from build123d import *

# Parameters (mm, degrees)
SKETCH1_R           = 2.125
SKETCH1_R_2         = 3
SKETCH1_W           = 6.35
SKETCH1_H           = 6
SKETCH1_W_2         = 12.7
SKETCH1_H_2         = 5.9944
SKETCH1_H_3         = 6.35
BOSS_EXTRUDE1_DEPTH = 5.9944


with BuildPart() as part:
    # Sketch1 → Boss-Extrude1 (new body)
    with BuildSketch(Plane(origin=(0, 0, 0), x_dir=(-1, 0, 0), z_dir=(0, 0, 1))):
        with BuildLine():
            Line((70.702589937, 1.66614002), (72.098749997, 1.66614002))
            Line((72.098749997, 1.66614002), (72.098749997, 7.383354962))
            Line((72.098749997, 7.383354962), (65.748749997, 7.383354962))
            Line((65.748749997, 7.383354962), (65.748749997, 13.383354962))
            Line((65.748749997, 13.383354962), (72.098749997, 13.383354962))
            Line((72.098749997, 13.383354962), (72.098749997, 45.072109768))
            ThreePointArc((72.098749997, 45.072109768), (69.866903669, 50.460263441), (64.478749997, 52.692109768))
            Line((64.478749997, 52.692109768), (45.302589937, 52.692109768))
            Line((45.302589937, 52.692109768), (19.902589937, 52.692109768))
            Line((19.902589937, 52.692109768), (-35.623445702, 52.692109768))
            ThreePointArc((-35.623445702, 52.692109768), (-40.113573763, 50.832237829), (-41.973445702, 46.342109768))
            Line((-41.973445702, 46.342109768), (-41.973445702, -49.004229729))
            ThreePointArc((-41.973445702, -49.004229729), (-40.113573763, -53.494357789), (-35.623445702, -55.354229729))
            Line((-35.623445702, -55.354229729), (19.902589937, -55.354229729))
            Line((19.902589937, -55.354229729), (45.302589937, -55.354229729))
            Line((45.302589937, -55.354229729), (64.478749997, -55.354229729))
            ThreePointArc((64.478749997, -55.354229729), (69.866903669, -53.122383402), (72.098749997, -47.734229729))
            Line((72.098749997, -47.734229729), (72.098749997, -12.840645038))
            Line((72.098749997, -12.840645038), (65.748749997, -12.840645038))
            Line((65.748749997, -12.840645038), (65.748749997, -6.840645038))
            Line((65.748749997, -6.840645038), (72.098749997, -6.840645038))
            Line((72.098749997, -6.840645038), (72.098749997, -4.32825998))
            Line((72.098749997, -4.32825998), (70.702589937, -4.32825998))
            Line((70.702589937, -4.32825998), (65.829579937, -4.32825998))
            Line((65.829579937, -4.32825998), (65.829579937, 1.66614002))
            Line((65.829579937, 1.66614002), (70.702589937, 1.66614002))
        make_face()
        with Locations((-10.170420063, -18.840645038)):
            Circle(SKETCH1_R, mode=Mode.SUBTRACT)
        with Locations((66.848749997, -36.840645038)):
            Circle(SKETCH1_R, mode=Mode.SUBTRACT)
        with Locations((42.848749997, -18.840645038)):
            Circle(SKETCH1_R, mode=Mode.SUBTRACT)
        with Locations((-28.770420063, -43.34064498)):
            Circle(SKETCH1_R_2, mode=Mode.SUBTRACT)
        with Locations((-28.770420063, -12.34064498)):
            Circle(SKETCH1_R_2, mode=Mode.SUBTRACT)
        with Locations((13.829579937, -18.840645038)):
            Circle(SKETCH1_R, mode=Mode.SUBTRACT)
        with Locations((42.848749997, -36.840645038)):
            Circle(SKETCH1_R, mode=Mode.SUBTRACT)
        with Locations((-10.170420063, -36.840645038)):
            Circle(SKETCH1_R, mode=Mode.SUBTRACT)
        with Locations((66.848749997, -18.840645038)):
            Circle(SKETCH1_R, mode=Mode.SUBTRACT)
        with Locations((13.829579937, -36.840645038)):
            Circle(SKETCH1_R, mode=Mode.SUBTRACT)
        with Locations((-28.770420063, 9.67852502)):
            Circle(SKETCH1_R_2, mode=Mode.SUBTRACT)
        with Locations((-28.770420063, 40.67852502)):
            Circle(SKETCH1_R_2, mode=Mode.SUBTRACT)
        with Locations((-10.170420063, 34.178525078)):
            Circle(SKETCH1_R, mode=Mode.SUBTRACT)
        with Locations((13.829579937, 34.178525078)):
            Circle(SKETCH1_R, mode=Mode.SUBTRACT)
        with Locations((13.829579937, 16.178525078)):
            Circle(SKETCH1_R, mode=Mode.SUBTRACT)
        with Locations((-10.170420063, 16.178525078)):
            Circle(SKETCH1_R, mode=Mode.SUBTRACT)
        with Locations((42.848749997, 34.178525078)):
            Circle(SKETCH1_R, mode=Mode.SUBTRACT)
        with Locations((66.848749997, 34.178525078)):
            Circle(SKETCH1_R, mode=Mode.SUBTRACT)
        with Locations((66.848749997, 16.178525078)):
            Circle(SKETCH1_R, mode=Mode.SUBTRACT)
        with Locations((42.848749997, 16.178525078)):
            Circle(SKETCH1_R, mode=Mode.SUBTRACT)
        with Locations((49.873749997, 10.383354962)):
            Rectangle(SKETCH1_W, SKETCH1_H, mode=Mode.SUBTRACT)
        with Locations((-29.420420063, -1.33105998)):
            Rectangle(SKETCH1_W_2, SKETCH1_H_2, mode=Mode.SUBTRACT)
        with Locations((49.873749997, -9.840645038)):
            Rectangle(SKETCH1_W, SKETCH1_H, mode=Mode.SUBTRACT)
        with Locations((-4.020420063, -1.33105998)):
            Rectangle(SKETCH1_W_2, SKETCH1_H_2, mode=Mode.SUBTRACT)
        with Locations((21.379579937, -1.33105998)):
            Rectangle(SKETCH1_W_2, SKETCH1_H_2, mode=Mode.SUBTRACT)
        with Locations((46.779579937, -1.33105998)):
            Rectangle(SKETCH1_W_2, SKETCH1_H_2, mode=Mode.SUBTRACT)
        with Locations((18.204579937, 5.84394002)):
            Rectangle(SKETCH1_W, SKETCH1_H_3, mode=Mode.SUBTRACT)
        with Locations((37.254579937, -8.50605998)):
            Rectangle(SKETCH1_W, SKETCH1_H_3, mode=Mode.SUBTRACT)
        with Locations((18.204579937, -8.50605998)):
            Rectangle(SKETCH1_W, SKETCH1_H_3, mode=Mode.SUBTRACT)
        with Locations((37.254579937, 5.84394002)):
            Rectangle(SKETCH1_W, SKETCH1_H_3, mode=Mode.SUBTRACT)
    extrude(amount=BOSS_EXTRUDE1_DEPTH)


solid = part.part
Geometry check sheet. Reference: the model listing, model coordinates, mm. A direction names the side the tool comes from. Round coordinates to 2 decimals unless told otherwise and drop trailing zeros. Write each loop counter-clockwise with the first axis right and the second up, starting at its lowest first coordinate (ties: lowest second). Pieces come first, ordered by that corner, then holes.
Item 1: Section check C-C (x = -49.5). Record the boundary of the cut face in (y, z), plus the area to 3 significant figures.
Determined:
outline: (-52.69, 0) - (-13.38, 0) - (-13.38, 5.99) - (-52.69, 5.99) - close; (-7.38, 0) - (-1.67, 0) - (-1.67, 5.99) - (-7.38, 5.99) - close; (4.33, 0) - (6.84, 0) - (6.84, 5.99) - (4.33, 5.99) - close; (12.84, 0) - (55.35, 0) - (55.35, 5.99) - (12.84, 5.99) - close
area: 540 mm2
Item 2: Section check A-A (x = 6). Record the boundary of the cut face in (y, z), plus the area to 3 significant figures.
Determined:
outline: (-52.69, 0) - (-1.67, 0) - (-1.67, 5.99) - (-52.69, 5.99) - close; (4.33, 0) - (55.35, 0) - (55.35, 5.99) - (4.33, 5.99) - close
area: 612 mm2
Item 3: Material ranges on line 1 along X through (y, z) = (-34, 4.75); line 2 along Y through (x, z) = (28.5, 4.7); line 3 along X through (y, z) = (8.5, 5.75), recorded low to high.
Determined:
line 1: x = -72.1 to -68.97, -64.73 to -44.97, -40.73 to -15.95, -11.71 to 8.05, 12.29 to 41.97
line 2: y = -52.69 to -43.67, -37.69 to -12.67, -6.69 to -1.67, 4.33 to 9.35, 15.33 to 40.35, 46.33 to 55.35
line 3: x = -65.75 to -53.05, -46.7 to -40.43, -34.08 to -21.38, -15.03 to 41.97
Item 4: Go/stop test with a flat-tipped pin: pin 1 Ø7 at (x, y) = (28.77, -9.68) entering from +Z. Record where the tip stops, or that it passes through.
Determined:
pin 1: stops at z = 5.99
Item 5: Mould release check, pull along Y, two halves, no side actions. Record for faces 3 (the face through (-18, 5.331, 3)), 4 (the face through (-14, 1, 0)), 5 (the face through (-69.926, -50.401, 2.955)), 6 (the face through (-18, -9.019, 3)): +Y half, -Y half, draft (parallel to the pull), parting line (faces both ways), or undercut.
Determined:
face 3: undercut
face 4: draft
face 5: -Y half
face 6: undercut
Item 6: Access from +Z, -Z, +X, -X, +Y, -Y to the whole of each face (thin tool, end or side, straight path). Record for faces 1 (the face through (-15.03, -6, 3)), 2 (the face through (-69, -7.383, 3)).
Determined:
face 1: +Z, -Z
face 2: +Z, -Z, -X
Item 7: Section check B-B (x = -20). Record the boundary of the cut face in (y, z).
Determined:
outline: (-52.69, 0) - (-9.02, 0) - (-9.02, 5.99) - (-52.69, 5.99) - close; (-2.67, 0) - (-1.67, 0) - (-1.67, 5.99) - (-2.67, 5.99) - close; (4.33, 0) - (5.33, 0) - (5.33, 5.99) - (4.33, 5.99) - close; (11.68, 0) - (55.35, 0) - (55.35, 5.99) - (11.68, 5.99) - close
Item 8: Section check D-D (z = 3.3). Give the number of separate pieces and of enclosed holes in the cut face, plus the area to 3 significant figures.
Determined:
separate pieces: 1
enclosed holes: 30
area: 11,300 mm2
